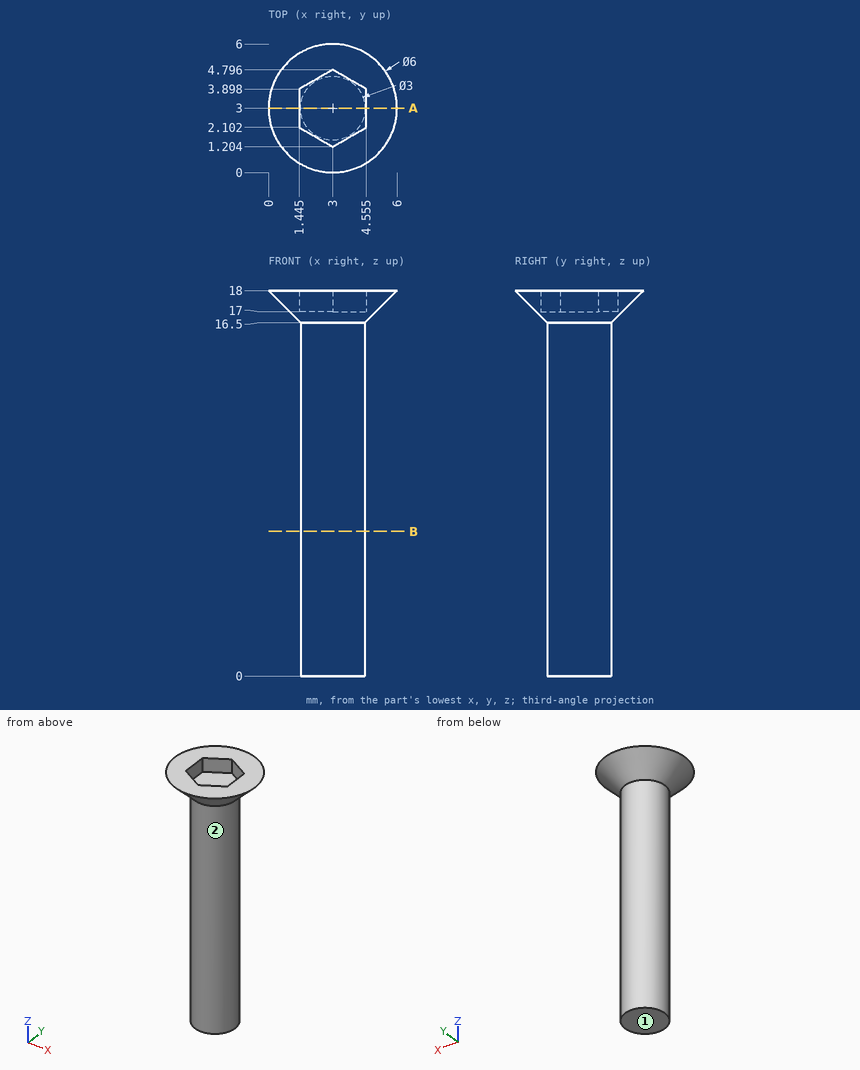
Part print with two shaded views. Sizes in mm from the minimum x, y, z corner. A direction names the side the tool comes from. Coordinates: 2 decimals unless noted, no trailing zeros. Write each loop counter-clockwise with the first axis right and the second up, starting at its lowest first coordinate (ties: lowest second). Pieces come first, ordered by that corner, then holes.
(1) Cut at B-B on z = 6.75. List the corners of the cut face in (x, y).
(2) Cut at A-A on y = 3. List the corners of the cut face in (x, z) (1 decimal).
(3) Pin check, flat tips, straight feed: pin 1 Ø3 at (x, z) = (5, 14.5) entering from -Y (1 decimal); pin 2 Ø1.5 at (x, z) = (3.5, 9.5) entering from +Y; pin 3 Ø0.5 at (y, z) = (3, 17.5) entering from +X. Stop position of each tip, or through.
(4) Drill centre lines: line 1 (Z direction, x = 3.15, y = 1.55); line 2 (X direction, y = 2.9, z = 1.5); line 3 (Y direction, x = 3.95, z = 8.5). Where is each one in solid material? Low to high.
(5) 3-axis set-ups, long thin cutter, end or side, ignore diameter. For the marked faces 1 and 2: which of +Z, -Z, +X, -X, +Y, -Y reach the whole face in a straight line?
Working result:
1. outline: circle Ø3 at (3, 3)
2. outline: (0, 18) - (1.5, 16.5) - (1.5, 0) - (4.5, 0) - (4.5, 16.5) - (6, 18) - (4.6, 18) - (4.6, 17) - (1.4, 17) - (1.4, 18) - close
3. pin 1: stops at y = 1.6
3. pin 2: stops at y = 4.5
3. pin 3: stops at x = 5.75
4. line 1: z = 0 to 17
4. line 2: x = 1.5 to 4.5
4. line 3: y = 1.84 to 4.16
5. face 1: -Z, +X, -X, +Y, -Y
5. face 2: -Z
